from build123d import *

# Parameters (mm, degrees)
SKETCH1_W                             = 98
SKETCH1_H                             = 95
BOSS_EXTRUDE1_DEPTH                   = 5
SKETCH6_W                             = 5
SKETCH6_H                             = 95
CUT_EXTRUDE1_DEPTH                    = 3
CUT_EXTRUDE2_DEPTH                    = 6
TAP_DRILL_FOR_M2X0_4_TAP4_D           = 2
TAP_DRILL_FOR_M2X0_4_TAP1_D           = 2
TAP_DRILL_FOR_M2X0_4_TAP1_CSINK_D     = 4.2
TAP_DRILL_FOR_M2X0_4_TAP1_CSINK_ANGLE = 90
TAP_DRILL_FOR_M2X0_4_TAP3_D           = 2
TAP_DRILL_FOR_M2X0_4_TAP3_DEPTH       = 6
TAP_DRILL_FOR_M2X0_4_TAP3_TIP         = 0.600860619
TAP_DRILL_FOR_M2X0_4_TAP5_D           = 2
TAP_DRILL_FOR_M2X0_4_TAP5_DEPTH       = 4
TAP_DRILL_FOR_M2X0_4_TAP5_TIP         = 0.600860619
TAP_DRILL_FOR_M2X0_4_TAP6_D           = 2
TAP_DRILL_FOR_M2X0_4_TAP6_DEPTH       = 7
TAP_DRILL_FOR_M2X0_4_TAP6_TIP         = 0.600860619


with BuildPart() as part:
    # Sketch1 → Boss-Extrude1 (new body)
    with BuildSketch(Plane(origin=(0, 0, 0), x_dir=(1, 0, 0), z_dir=(0, 1, 0))):
        with Locations((49, 47.5)):
            Rectangle(SKETCH1_W, SKETCH1_H)
    extrude(amount=BOSS_EXTRUDE1_DEPTH)

    # Sketch6 → Cut-Extrude1 (cut)
    with BuildSketch(Plane(origin=(0, 5, 0), x_dir=(1, 0, 0), z_dir=(0, 1, 0))):
        with Locations((2.5, 47.5)):
            Rectangle(SKETCH6_W, SKETCH6_H)
    extrude(amount=-CUT_EXTRUDE1_DEPTH, mode=Mode.SUBTRACT)

    # Sketch5 → Cut-Extrude2 (cut, through all)
    with BuildSketch(Plane(origin=(0, 5, 0), x_dir=(1, 0, 0), z_dir=(0, 1, 0))):
        with BuildLine():
            Line((15, 90), (40, 90))
            ThreePointArc((40, 90), (43.535533906, 88.535533906), (45, 85))
            Line((45, 85), (45, 50))
            ThreePointArc((45, 50), (43.535533906, 46.464466094), (40, 45))
            Line((40, 45), (15, 45))
            ThreePointArc((15, 45), (11.464466094, 46.464466094), (10, 50))
            Line((10, 50), (10, 85))
            ThreePointArc((10, 85), (11.464466094, 88.535533906), (15, 90))
        make_face()
        with BuildLine():
            Line((60, 90), (85, 90))
            ThreePointArc((85, 90), (88.535533906, 88.535533906), (90, 85))
            Line((90, 85), (90, 50))
            ThreePointArc((90, 50), (88.535533906, 46.464466094), (85, 45))
            Line((85, 45), (60, 45))
            ThreePointArc((60, 45), (56.464466094, 46.464466094), (55, 50))
            Line((55, 50), (55, 85))
            ThreePointArc((55, 85), (56.464466094, 88.535533906), (60, 90))
        make_face()
        with BuildLine():
            Line((60, 35), (85, 35))
            ThreePointArc((85, 35), (88.535533906, 33.535533906), (90, 30))
            Line((90, 30), (90, 15))
            ThreePointArc((90, 15), (88.535533906, 11.464466094), (85, 10))
            Line((85, 10), (60, 10))
            ThreePointArc((60, 10), (56.464466094, 11.464466094), (55, 15))
            Line((55, 15), (55, 30))
            ThreePointArc((55, 30), (56.464466094, 33.535533906), (60, 35))
        make_face()
        with BuildLine():
            Line((15, 35), (40, 35))
            ThreePointArc((40, 35), (43.535533906, 33.535533906), (45, 30))
            Line((45, 30), (45, 15))
            ThreePointArc((45, 15), (43.535533906, 11.464466094), (40, 10))
            Line((40, 10), (15, 10))
            ThreePointArc((15, 10), (11.464466094, 11.464466094), (10, 15))
            Line((10, 15), (10, 30))
            ThreePointArc((10, 30), (11.464466094, 33.535533906), (15, 35))
        make_face()
    extrude(amount=-CUT_EXTRUDE2_DEPTH, mode=Mode.SUBTRACT)

    # Tap Drill for M2x0.4 Tap4 (through all)
    with Locations(Plane(origin=(22.568, 5, -40), x_dir=(0, 0, 1), z_dir=(0, 1, 0))):
        with Locations((0, 0), (0, 54.864)):
            Hole(TAP_DRILL_FOR_M2X0_4_TAP4_D / 2)

    # Tap Drill for M2x0.4 Tap1 (through all)
    with Locations(Plane(origin=(2.5, 0, -15), x_dir=(0, 0, -1), z_dir=(0, -1, 0))):
        with Locations((0, 0), (70, 0)):
            CounterSinkHole(TAP_DRILL_FOR_M2X0_4_TAP1_D / 2, TAP_DRILL_FOR_M2X0_4_TAP1_CSINK_D / 2, counter_sink_angle=TAP_DRILL_FOR_M2X0_4_TAP1_CSINK_ANGLE)

    # Tap Drill for M2x0.4 Tap3
    with Locations(Plane(origin=(98, 2.5, -15), x_dir=(0, 0, 1), z_dir=(1, 0, 0))):
        with Locations((0, 0), (-70, 0)):
            Hole(TAP_DRILL_FOR_M2X0_4_TAP3_D / 2, depth=TAP_DRILL_FOR_M2X0_4_TAP3_DEPTH)
            with Locations((0, 0, -(TAP_DRILL_FOR_M2X0_4_TAP3_DEPTH + TAP_DRILL_FOR_M2X0_4_TAP3_TIP / 2))):  # 118° drill point
                Cone(0, TAP_DRILL_FOR_M2X0_4_TAP3_D / 2, TAP_DRILL_FOR_M2X0_4_TAP3_TIP, mode=Mode.SUBTRACT)

    # Tap Drill for M2x0.4 Tap5
    with Locations(Plane(origin=(92.75, 2.5, -95), x_dir=(-1, 0, 0), z_dir=(0, 0, -1))):
        with Locations((0, 0), (85.5, 0)):
            Hole(TAP_DRILL_FOR_M2X0_4_TAP5_D / 2, depth=TAP_DRILL_FOR_M2X0_4_TAP5_DEPTH)
            with Locations((0, 0, -(TAP_DRILL_FOR_M2X0_4_TAP5_DEPTH + TAP_DRILL_FOR_M2X0_4_TAP5_TIP / 2))):  # 118° drill point
                Cone(0, TAP_DRILL_FOR_M2X0_4_TAP5_D / 2, TAP_DRILL_FOR_M2X0_4_TAP5_TIP, mode=Mode.SUBTRACT)

    # Tap Drill for M2x0.4 Tap6
    with Locations(Plane(origin=(25, 2.5, 0), x_dir=(1, 0, 0), z_dir=(0, 0, 1))):
        with Locations((0, 0), (50, 0)):
            Hole(TAP_DRILL_FOR_M2X0_4_TAP6_D / 2, depth=TAP_DRILL_FOR_M2X0_4_TAP6_DEPTH)
            with Locations((0, 0, -(TAP_DRILL_FOR_M2X0_4_TAP6_DEPTH + TAP_DRILL_FOR_M2X0_4_TAP6_TIP / 2))):  # 118° drill point
                Cone(0, TAP_DRILL_FOR_M2X0_4_TAP6_D / 2, TAP_DRILL_FOR_M2X0_4_TAP6_TIP, mode=Mode.SUBTRACT)


solid = part.part
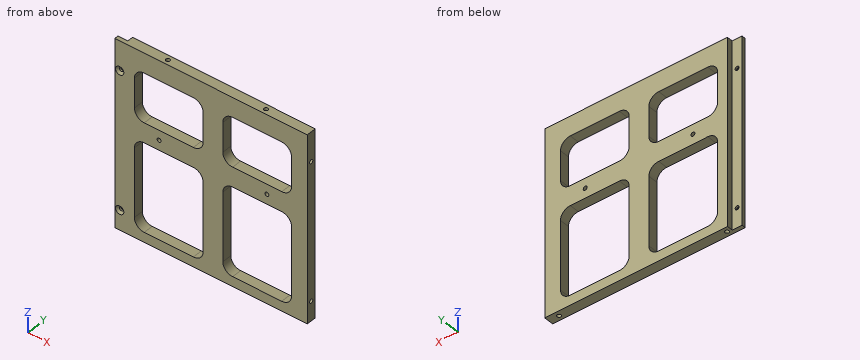
Input: part model. Units: mm. Frame: model coordinates. Round coordinates to 2 decimals unless told otherwise and drop trailing zeros. Write each loop counter-clockwise with the first axis right and the second up, starting at its lowest first coordinate (ties: lowest second). Pieces come first, ordered by that corner, then holes.
1) Cut plane A-A (z = -65). Return the cut outline in (x, y), then the cut area to 3 significant figures.
2) Contact query for flat-ended pins moving along their axis: P1, Ø1.8, axis at x = 77.432, z = -40, coming from the +Y side; P2, Ø1.8, axis at x = 75, y = 2.5, coming from the +Z side. Output: stop coordinate, or through.
3) Ray query, L1, parallel to X at y = 1.4, z = -15; L2, parallel to Z at x = 75.5, y = 4.65; L3, parallel to Z at x = 2.5, y = 1.6. Return the intervals inside material, ascending.
4) Cut plane B-B (x = 83.5). Return the cut outline in (y, z).
Geometry says:
1. outline: (0, 0) - (10, 0) - (10, 5) - (5, 5) - (5, 2) - (0, 2) - close; (45, 0) - (55, 0) - (55, 5) - (45, 5) - close; (90, 0) - (98, 0) - (98, 5) - (90, 5) - close
1. area: 125 mm2
2. P1: passes through
2. P2: stops at z = -7.06
3. L1: x = 0 to 1.5, 3.5 to 10, 45 to 55, 90 to 98
3. L2: z = -95 to -90, -45 to -35, -10 to 0
3. L3: z = -95 to -86, -84 to -16, -14 to 0
4. outline: (0, -95) - (5, -95) - (5, -90) - (0, -90) - close; (0, -45) - (5, -45) - (5, -35) - (0, -35) - close; (0, -10) - (5, -10) - (5, 0) - (0, 0) - close
